```python
from build123d import *

# Parameters (mm, degrees)
ESQUISSE1_W             = 44
ESQUISSE1_H             = 34
BOSS_EXTRU_1_DEPTH      = 14
COQUE1_T                = -1.5
ESQUISSE2_W             = 1.5
ESQUISSE2_H             = 13
ENL_V_MAT_EXTRU_1_DEPTH = 10


with BuildPart() as part:
    # Esquisse1 → Boss.-Extru.1 (new body)
    with BuildSketch(Plane(origin=(0, 0, 0), x_dir=(1, 0, 0), z_dir=(0, 1, 0))):
        Rectangle(ESQUISSE1_W, ESQUISSE1_H)
    extrude(amount=BOSS_EXTRU_1_DEPTH)

    # Coque1
    coque1_openings = [part.faces().sort_by_distance(p)[0] for p in [
        (0, 14, 0),
    ]]
    offset(amount=COQUE1_T, openings=coque1_openings, kind=Kind.INTERSECTION)

    # Esquisse2 → Enlèv. mat.-Extru.1 (cut)
    with BuildSketch(Plane(origin=(0, 14, 0), x_dir=(1, 0, 0), z_dir=(0, 1, 0))):
        with Locations((21.25, 0)):
            Rectangle(ESQUISSE2_W, ESQUISSE2_H)
    extrude(amount=-ENL_V_MAT_EXTRU_1_DEPTH, mode=Mode.SUBTRACT)


solid = part.part
```
For this review, take the finished solid that the model builds, in its own axes (mm). A direction names the side the tool comes from. Coordinates: 2 decimals unless noted, no trailing zeros. Order: outer loops, then holes, each group sorted by start corner. A loop starts at its lowest first (then second) coordinate and runs counter-clockwise, first axis right, second up. Notation, with made-up numbers: (34.5, 74.5) -> (80.5, 74.5) arc R30 ccw to (80.5, 105.5) -> close; hole circle Ø10 at (87, 60.5). An arc over 180 degrees is marked (long way). Use CSV: the item, a comma, the result in double quotes. Start each with the question number.
Item 1: Wall thickness on probe 1 along X at (y, z) = (4.5, 13.5); probe 2 along Z at (x, y) = (14.5, 9); probe 3 along Y at (x, z) = (5, -14): over which ranges is each line inside the solid? List them lowest first.
Item 2: We need section A-A, the plane y = 3.25. Give the boundary of the cut face in (x, z).
Item 3: We need section B-B, the plane z = 2. Give the boundary of the cut face in (x, y).
Item 4: We need section C-C, the plane y = 9.75. Give the boundary of the cut face in (x, z), then the cut area to 4 significant figures.
Item 5: For faces 5 (the face through (20.5, 3, 0)), 6 (the face through (0, 7, 17)), 7 (the face through (21, 9, -6.5)), list the 3-axis set-ups (+Z, -Z, +X, -X, +Y, -Y) from which the entire face can be reached by the end or side of a thin tool; tool diameter is ignored.
Item 6: Insertion check: pin 1 (15.5 mm diameter, centred on x = -0.5, z = 0.5, fed in from +Y); pin 2 (1.6 mm diameter, centred on x = 21, z = -2.5, fed in from +Y). Each pin has a flat end and moves straight along its axis. Give the tip position at first contact, or say it passes through.
Item 7: Draft analysis for pull direction X (two halves, no side actions). For faces 1 (the face through (22, 3.8, 0.2)), 2 (the face through (-20.5, 8, 0)), 3 (the face through (21, 9, 6.5)), 4 (the face through (-22, 7, 0)), state which applies: pulls with the +X half, pulls with the -X half, needs draft (parallel to the pull), parting line crosses it, or undercut.
Item 8: We need section D-D, the plane x = -12.5. Give the boundary of the cut face in (y, z), then the cut area to 3 significant figures.
Derived:
1,probe 1,"x = -22 to -20.5, 20.5 to 22"
1,probe 2,"z = -17 to -15.5, 15.5 to 17"
1,probe 3,"y = 0 to 1.5"
2,outline,"(-22, -17) -> (22, -17) -> (22, 17) -> (-22, 17) -> close; hole (-20.5, -15.5) -> (20.5, -15.5) -> (20.5, 15.5) -> (-20.5, 15.5) -> close"
3,outline,"(-22, 0) -> (22, 0) -> (22, 4) -> (20.5, 4) -> (20.5, 1.5) -> (-20.5, 1.5) -> (-20.5, 14) -> (-22, 14) -> close"
4,outline,"(-22, -17) -> (22, -17) -> (22, -6.5) -> (20.5, -6.5) -> (20.5, -15.5) -> (-20.5, -15.5) -> (-20.5, 15.5) -> (20.5, 15.5) -> (20.5, 6.5) -> (22, 6.5) -> (22, 17) -> (-22, 17) -> close"
4,area,"205.5 mm^2"
5,face 5,"+Y"
5,face 6,"+Z, +X, -X, +Y, -Y"
5,face 7,"+X, +Y"
6,pin 1,"stops at y = 1.5"
6,pin 2,"stops at y = 4"
7,face 1,"pulls with the +X half"
7,face 2,"undercut"
7,face 3,"needs draft"
7,face 4,"pulls with the -X half"
8,outline,"(0, -17) -> (14, -17) -> (14, -15.5) -> (1.5, -15.5) -> (1.5, 15.5) -> (14, 15.5) -> (14, 17) -> (0, 17) -> close"
8,area,"88.5 mm^2"
